Geometry: final body of the model. Coordinates: model frame, mm. A direction names the side the tool comes from. Coordinates: 2 decimals unless noted, no trailing zeros. Loops run counter-clockwise (first coordinate to the right, second up) from the corner with the lowest first, then second, coordinate; pieces in that order, holes last. Notation, with made-up numbers: (62.25, 82.25) -> (118.25, 82.25) arc R21 cw to (118.25, 93.25) -> close; hole circle Ø3 at (18, 23). An arc over 180 degrees is marked (long way). One line per item, written item: value. Start each with the question number.
from build123d import *

# Parameters (mm, degrees)
RACCORDO1_R                  = 20
ESTRUSIONE_ESTRUSIONE1_START = 1
ESTRUSIONE_ESTRUSIONE1_DEPTH = 1


with BuildPart() as part:
    # Schizzo1 → Rivoluzione1 (revolve)
    with BuildSketch(Plane.XY, mode=Mode.PRIVATE) as rivoluzione1_sk:
        Polygon((-35, 99), (35, 99), (35, 10), (15.51, 10), (15.51, 17.5), (4.51, 17.5), (4.51, 32.5), (-28.39, 32.5), (-28.39, 56.75), (-35, 56.75), align=None)
    revolve(rivoluzione1_sk.sketch.rotate(Axis((45, 0, 0), (-1, 0, 0)), 90), axis=Axis((45, 0, 0), (-1, 0, 0)))

    # Raccordo1
    raccordo1_edges = [part.edges().sort_by_distance(p)[0] for p in [
        (35, 0, 99),
        (-35, 0, 99),
    ]]
    fillet(raccordo1_edges, radius=RACCORDO1_R)

    # Schizzo2 → Estrusione-Estrusione1 (add)
    with BuildSketch(Plane.ZY.offset(35).offset(ESTRUSIONE_ESTRUSIONE1_START)):
        with BuildLine():
            Line((-5, 66.529306559), (5, 66.529306559))
            Line((5, 66.529306559), (5, 56.529306559))
            ThreePointArc((5, 56.529306559), (0, 56.75), (-5, 56.529306559))
            Line((-5, 56.529306559), (-5, 66.529306559))
        make_face()
    extrude(amount=-ESTRUSIONE_ESTRUSIONE1_DEPTH)


solid = part.part
1. Draft query along Y for faces 1 (the face through (9.933, 17.084, 3.794)), 2 (the face through (-35, -19, -54)), 3 (the face through (0.21, -66.909, 72.967)). Return one class per face: released by +Y, released by -Y, zero draft, split by the parting line, or undercut.
2. Pin query (flat end, axial travel): pin 1 Ø1 at (x, y) = (-16.5, -43.5) entering from -Z; pin 2 Ø10 at (x, z) = (26, 45) entering from +Y; pin 3 Ø12 at (y, z) = (45.5, -13) entering from -X. Return the tip coordinate at first contact, or that it passes through.
3. Set-up query: faces 4 (the face through (35, 16, 1)), 5 (the face through (4.51, 14, 14)). Return all of +Z, -Z, +X, -X, +Y, -Y with unobstructed straight access to the full face (end or side cutting, diameter ignored); none if empty.
4. Line query: L1, parallel to Y at x = 12, z = 0; L2, parallel to X at y = -64.5, z = 35; L3, parallel to Y at x = -25, z = 9. Output: solid intervals per line, ascending. Write a range as [from, to].
5. Section C-C on x = 24.5. Return the cut outline in (y, z).
6. Section D-D on x = -24.5. Return the cut outline in (y, z).
7. Section B-B on z = 0. Return the cut outline in (x, y).
8. Section A-A on y = 0. Return the cut outline in (x, z), plus the area to 3 significant figures.
Checks:
1. face 1: undercut
1. face 2: zero draft
1. face 3: split by the parting line
2. pin 1: z = -89.11
2. pin 2: y = 88.31
2. pin 3: x = -28.39
3. face 4: +Z, -Z, +X, +Y, -Y
3. face 5: -X
4. L1: [-99, -17.5], [17.5, 99]
4. L2: [-35, 35]
4. L3: [-95.9, -31.23], [31.23, 95.9]
5. outline: circle Ø193.2 at (0, 0); hole circle Ø20 at (0, 0)
6. outline: circle Ø193.2 at (0, 0); hole circle Ø65 at (0, 0)
7. outline: (-36, 56.75) -> (-28.39, 56.75) -> (-28.39, 32.5) -> (4.51, 32.5) -> (4.51, 17.5) -> (15.51, 17.5) -> (15.51, 10) -> (35, 10) -> (35, 79) arc R20 ccw to (15, 99) -> (-15, 99) arc R20 ccw to (-35, 79) -> (-35, 66.53) -> (-36, 66.53) -> close; (-35, -79) arc R20 ccw to (-15, -99) -> (15, -99) arc R20 ccw to (35, -79) -> (35, -10) -> (15.51, -10) -> (15.51, -17.5) -> (4.51, -17.5) -> (4.51, -32.5) -> (-28.39, -32.5) -> (-28.39, -56.75) -> (-35, -56.75) -> close
8. outline: (-35, -79) arc R20 ccw to (-15, -99) -> (15, -99) arc R20 ccw to (35, -79) -> (35, -10) -> (15.51, -10) -> (15.51, -17.5) -> (4.51, -17.5) -> (4.51, -32.5) -> (-28.39, -32.5) -> (-28.39, -56.75) -> (-35, -56.75) -> close; (-35, 56.75) -> (-28.39, 56.75) -> (-28.39, 32.5) -> (4.51, 32.5) -> (4.51, 17.5) -> (15.51, 17.5) -> (15.51, 10) -> (35, 10) -> (35, 79) arc R20 ccw to (15, 99) -> (-15, 99) arc R20 ccw to (-35, 79) -> close
8. area: 9,850 mm²
